Could you check a few things on this drawing? It's one solid part, dimensions in mm from its lowest x, y, z. A direction names the side the tool comes from. Give positions to 0.01 mm unless a question says otherwise; leave off trailing zeros. Order: outer loops, then holes, each group sorted by start corner. A loop starts at its lowest first (then second) coordinate and runs counter-clockwise, first axis right, second up. Notation, with made-up numbers: (-4, 32.25) -> (5, 32.25) arc R24 cw to (5, 51.25) -> close; hole circle Ø2 at (30, 59.25). An arc over 180 degrees is marked (long way). Answer as a JSON object with one key per item and string values.
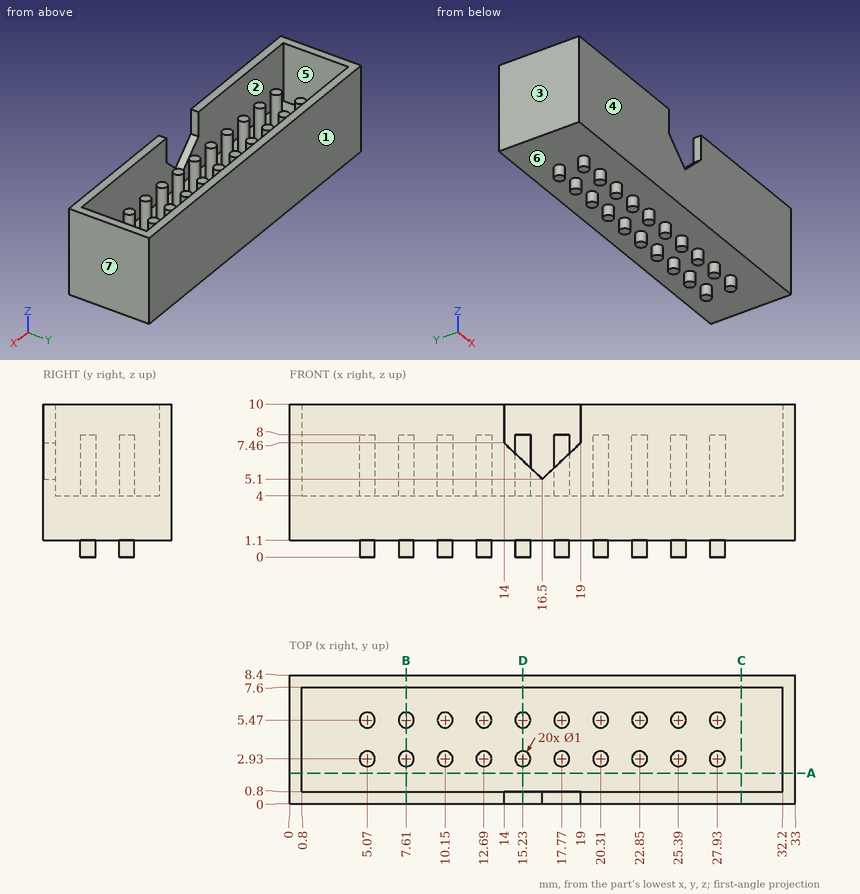
1. Will these pins go through, and if not, where does the flat tip stop? pin 1 Ø0.6 at (y, z) = (0.5, 8) entering from -X; pin 2 Ø0.8 at (x, y) = (5, 3) entering from +Z.
Worked answers:
{"pin 1": "x = 0", "pin 2": "z = 8"}
2. If we section it at A-A on y = 2: Please give me the cut outline in (x, z).
Worked answers:
{"outline": "(0, 1.1) -> (33, 1.1) -> (33, 10) -> (32.2, 10) -> (32.2, 4) -> (0.8, 4) -> (0.8, 10) -> (0, 10) -> close"}
3. For the marked faces 5, 6 and 7, which set-ups out of +Z, -Z, +X, -X, +Y, -Y let a thin tool reach every point of the face, with its end or its side?
Worked answers:
{"face 5": "+Z", "face 6": "-Z", "face 7": "+Z, -Z, +X, +Y, -Y"}
4. Please list where these lines run through material, in increasing order: L1, parallel to Y at x = 14.5, z = 5.5; L2, parallel to Y at x = 8, z = 7; L3, parallel to X at y = 4.25, z = 8.75.
Worked answers:
{"L1": "0 to 0.8, 7.6 to 8.4", "L2": "0 to 0.8, 2.62 to 3.24, 5.16 to 5.78, 7.6 to 8.4", "L3": "0 to 0.8, 32.2 to 33"}
5. If we section it at D-D on x = 15.23: Please give me the cut outline in (y, z).
Worked answers:
{"outline": "(0, 1.1) -> (2.43, 1.1) -> (2.43, 0) -> (3.43, 0) -> (3.43, 1.1) -> (4.97, 1.1) -> (4.97, 0) -> (5.97, 0) -> (5.97, 1.1) -> (8.4, 1.1) -> (8.4, 10) -> (7.6, 10) -> (7.6, 4) -> (5.97, 4) -> (5.97, 8) -> (4.97, 8) -> (4.97, 4) -> (3.43, 4) -> (3.43, 8) -> (2.43, 8) -> (2.43, 4) -> (0.8, 4) -> (0.8, 6.3) -> (0, 6.3) -> close"}
6. If we mould it in two halves opening along Y, with no side actions, what happens to the marked faces 1, 2, 3 and 4? For each: +Y half, -Y half, draft (parallel to the pull), parting line (faces both ways), or undercut.
Worked answers:
{"face 1": "+Y half", "face 2": "undercut", "face 3": "draft", "face 4": "-Y half"}
7. If we section it at B-B on x = 7.61: Please give me the cut outline in (y, z), then the cut area to 3 significant figures.
Worked answers:
{"outline": "(0, 1.1) -> (2.43, 1.1) -> (2.43, 0) -> (3.43, 0) -> (3.43, 1.1) -> (4.97, 1.1) -> (4.97, 0) -> (5.97, 0) -> (5.97, 1.1) -> (8.4, 1.1) -> (8.4, 10) -> (7.6, 10) -> (7.6, 4) -> (5.97, 4) -> (5.97, 8) -> (4.97, 8) -> (4.97, 4) -> (3.43, 4) -> (3.43, 8) -> (2.43, 8) -> (2.43, 4) -> (0.8, 4) -> (0.8, 10) -> (0, 10) -> close", "area": "44.2 mm²"}
8. If we section it at C-C on x = 29.5: Please give me the cut outline in (y, z), then the cut area to 3 significant figures.
Worked answers:
{"outline": "(0, 1.1) -> (8.4, 1.1) -> (8.4, 10) -> (7.6, 10) -> (7.6, 4) -> (0.8, 4) -> (0.8, 10) -> (0, 10) -> close", "area": "34.0 mm²"}
